from build123d import *

# Parameters (mm, degrees)
F0_R     = 5.55
F1_DEPTH = 5
F0_W     = 4.939636
F0_H     = 5.1
F2_DEPTH = 1
F3_W     = 4.9
F3_H     = 4.939636
F4_DEPTH = 4.8


with BuildPart() as f1:
    # F0 (on Top) → F1 (new body)
    with BuildSketch(Plane.XY):
        Circle(F0_R)
        with BuildLine():
            ThreePointArc((-2.469818, -2.55), (-3.55, 0), (-2.469818, 2.55))
            Line((-2.469818, 2.55), (2.469818, 2.55))
            ThreePointArc((2.469818, 2.55), (3.55, 0), (2.469818, -2.55))
            Line((2.469818, -2.55), (-2.469818, -2.55))
        make_face(mode=Mode.SUBTRACT)
    extrude(amount=F1_DEPTH)

    # F0 (on Top) → F2 (join)
    with BuildSketch(Plane.XY):
        Circle(F0_R)
        with BuildLine():
            ThreePointArc((-2.469818, -2.55), (-3.55, 0), (-2.469818, 2.55))
            Line((-2.469818, 2.55), (2.469818, 2.55))
            ThreePointArc((2.469818, 2.55), (3.55, 0), (2.469818, -2.55))
            Line((2.469818, -2.55), (-2.469818, -2.55))
        make_face(mode=Mode.SUBTRACT)
        with BuildLine():
            ThreePointArc((2.469818, -2.55), (3.55, 0), (2.469818, 2.55))
            Line((2.469818, 2.55), (2.469818, -2.55))
        make_face()
        Rectangle(F0_W, F0_H)
        with BuildLine():
            Line((-2.469818, -2.55), (-2.469818, 2.55))
            ThreePointArc((-2.469818, 2.55), (-3.55, 0), (-2.469818, -2.55))
        make_face()
    extrude(amount=-F2_DEPTH)

    # F3 (on face) → F4 (join)
    with BuildSketch(Plane(origin=(0, 0, -1), x_dir=(1, 0, 0), z_dir=(0, 0, -1))):
        Rectangle(F3_W, F3_H)
    extrude(amount=F4_DEPTH)


solid = f1.part
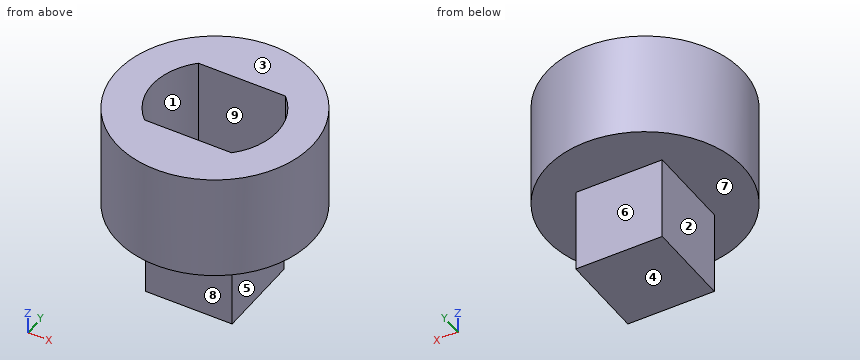
Could you check a few things on this model? Use its own coordinates, in mm. Face numbers are marked on the shaded views. A direction names the side the tool comes from. Round coordinates to 2 decimals unless told otherwise and drop trailing zeros. Write each loop counter-clockwise with the first axis right and the second up, starting at its lowest first coordinate (ties: lowest second). Pieces come first, ordered by that corner, then holes. Notation, with made-up numbers: (-31.5, -2) -> (-18.5, -2) arc R34 cw to (-18.5, 28) -> close; hole circle Ø11 at (54, 82.25). An arc over 180 degrees is marked (long way). Use a Markdown table: item, result.
1. If we section it at D-D (x = -3): List the corners of the cut face in (y, z) for me, then the cut area to 3 significant figures.
Answer key:
| item | result |
|---|---|
| outline | (-4.67, -1) -> (4.67, -1) -> (4.67, 5) -> (1.9, 5) -> (1.9, 0) -> (-1.9, 0) -> (-1.9, 5) -> (-4.67, 5) -> close |
| area | 37.1 mm^2 |
2. If we section it at C-C (x = 0): List the corners of the cut face in (y, z) for me.
Answer key:
| item | result |
|---|---|
| outline | (-5.55, -1) -> (-2.47, -1) -> (-2.47, -5.8) -> (2.47, -5.8) -> (2.47, -1) -> (5.55, -1) -> (5.55, 5) -> (2.55, 5) -> (2.55, 0) -> (-2.55, 0) -> (-2.55, 5) -> (-5.55, 5) -> close |
3. We'd pull the mould along Y, two halves only. Please class the marked faces 6, 7, 8 and 9: +Y half, -Y half, draft (parallel to the pull), parting line (faces both ways), or undercut.
Answer key:
| item | result |
|---|---|
| face 6 | +Y half |
| face 7 | draft |
| face 8 | -Y half |
| face 9 | undercut |
4. Which directions (+Z, -Z, +X, -X, +Y, -Y) give clear straight access to the entire face, cutting with the end or side of a thin tool? Please do the marked faces 1, 2, 3, 4 and 5.
Answer key:
| item | result |
|---|---|
| face 1 | +Z |
| face 2 | -Z, -X, +Y, -Y |
| face 3 | +Z, +X, -X, +Y, -Y |
| face 4 | -Z, +X, -X, +Y, -Y |
| face 5 | -Z, +X, +Y, -Y |
5. For pin 1 Ø2.5 at (x, y) = (1, 1) entering from +Z; pin 2 Ø1 at (y, z) = (2, -3.5) entering from +X; pin 3 Ø1.4 at (x, z) = (0, -2) entering from +Y, each with a flat end and sliding along its axis, tell me the tip position at first contact or that it passes through.
Answer key:
| item | result |
|---|---|
| pin 1 | stops at z = 0 |
| pin 2 | stops at x = 2.45 |
| pin 3 | stops at y = 2.47 |
6. Please list where these lines run through material, in increasing order: probe 1 along Z at (x, y) = (1, 2.5); probe 2 along Z at (x, y) = (-1.75, 1.75); probe 3 along X at (y, z) = (0, -4.25).
Answer key:
| item | result |
|---|---|
| probe 1 | z = -1 to 0 |
| probe 2 | z = -5.8 to 0 |
| probe 3 | x = -2.45 to 2.45 |
7. If we section it at A-A (y = 0): List the corners of the cut face in (x, z) for me, then the cut area to 3 significant figures.
Answer key:
| item | result |
|---|---|
| outline | (-5.55, -1) -> (-2.45, -1) -> (-2.45, -5.8) -> (2.45, -5.8) -> (2.45, -1) -> (5.55, -1) -> (5.55, 5) -> (3.55, 5) -> (3.55, 0) -> (-3.55, 0) -> (-3.55, 5) -> (-5.55, 5) -> close |
| area | 54.6 mm^2 |
8. If we section it at B-B (z = 4.5): List the corners of the cut face in (x, y) for me.
Answer key:
| item | result |
|---|---|
| outline | circle Ø11.1 at (0, 0); hole (-2.47, -2.55) -> (2.47, -2.55) arc R3.55 ccw to (2.47, 2.55) -> (-2.47, 2.55) arc R3.55 ccw to start |
